from build123d import *

# Parameters (mm, degrees)
BOSS_EXTRUDE1_DEPTH      = 49
CHAMFER1_SIZE            = 1
CHAMFER2_SIZE            = 1
SKETCH4_W                = 3.006754005
SKETCH4_H                = 49
BOSS_EXTRUDE2_DEPTH      = 5
SKETCH5_W                = 49
SKETCH5_H                = 5
BOSS_EXTRUDE3_DEPTH      = 6.139242
BOSS_EXTRUDE4_DEPTH      = 350
BOSS_EXTRUDE4_DEPTH_BACK = 70
SKETCH6_R                = 2.4
BOSS_EXTRUDE5_START      = 50
BOSS_EXTRUDE5_DEPTH      = 50
SKETCH11_R               = 0.5
BOSS_EXTRUDE9_DEPTH      = 2


with BuildPart() as part:
    # Sketch1 → Boss-Extrude1 (new body)
    with BuildSketch(Plane.XY):
        with BuildLine():
            Line((-6.350615501, -38.986147319), (-6.350615501, -41.01121411))
            ThreePointArc((-6.350615501, -41.01121411), (-1.360537007, -41.477692065), (3.649384499, -41.339230675))
            Line((3.649384499, -41.339230675), (3.649384499, -39.331056339))
            ThreePointArc((3.649384499, -39.331056339), (-1.361580989, -39.476525901), (-6.350615501, -38.986147319))
        make_face()
    extrude(amount=BOSS_EXTRUDE1_DEPTH)

    # Chamfer1
    # the kernel refuses this chamfer: 3, 1 mm, written as the material it takes off along each edge
    with BuildSketch(Plane(origin=(3.649384499, -41.339230675, -7.093753287), x_dir=(0, 1, 0), z_dir=(0, 0, 1))) as chamfer1_piece_1:
        with BuildLine():
            Line((CHAMFER1_SIZE, 0), (-0.150364113, 2.720124405))
            ThreePointArc((-0.150364113, 2.720124405), (-0.100586913, 1.415213895), (0, 0))
            Line((0, 0), (CHAMFER1_SIZE, 0))
        make_face()
    extrude(amount=63.187506575, mode=Mode.SUBTRACT)

    # Chamfer2
    # the kernel refuses this chamfer: 3, 1 mm, written as the material it takes off along each edge
    with BuildSketch(Plane(origin=(-6.350615501, -41.01121411, -7.077780992), x_dir=(0.992702552846142, -0.12058872904526673, 0), z_dir=(0, 0, 1))) as chamfer2_piece_1:
        with BuildLine():
            Line((2.717564067, 0), (-CHAMFER2_SIZE * 0.120588729045, CHAMFER2_SIZE * 0.992702552846))
            Line((-CHAMFER2_SIZE * 0.120588729045, CHAMFER2_SIZE * 0.992702552846), (0, 0))
            ThreePointArc((0, 0), (1.415420862, -0.022211756), (2.717564067, 0))
        make_face()
    extrude(amount=63.155561983, mode=Mode.SUBTRACT)

    # Sketch4 → Boss-Extrude2 (add)
    with BuildSketch(Plane(origin=(-17.090415502, -34.725548264, 0), x_dir=(0.8972243095002063, -0.44157506546665215, 0), z_dir=(-0.44157506546665215, -0.8972243095002063, 0))):
        with Locations((13.473404886, 24.5)):
            Rectangle(SKETCH4_W, SKETCH4_H)
    extrude(amount=BOSS_EXTRUDE2_DEPTH)

    # Sketch5 → Boss-Extrude3 (add)
    with BuildSketch(Plane(origin=(-12, 0, 0), x_dir=(0, 0, -1), z_dir=(1, 0, 0))):
        with Locations((-24.5, -45.003805325)):
            Rectangle(SKETCH5_W, SKETCH5_H)
    extrude(amount=BOSS_EXTRUDE3_DEPTH)

    # Sketch6 → Boss-Extrude4 (add, two sides: drawn at the far end of the back side and taken through both)
    with BuildSketch(Plane(origin=(0, 0, 0), x_dir=(-1, 0, 0), z_dir=(0, 0, -1)).offset(-BOSS_EXTRUDE4_DEPTH_BACK)):
        with Locations((12, -45.003805325)):
            Circle(SKETCH6_R)
    extrude(amount=BOSS_EXTRUDE4_DEPTH + BOSS_EXTRUDE4_DEPTH_BACK)

    # Sketch8 → Boss-Extrude5 (add)
    with BuildSketch(Plane(origin=(0, 0, -281.5), x_dir=(-1, 0, 0), z_dir=(0, 0, -1)).offset(BOSS_EXTRUDE5_START)):
        with BuildLine():
            Line((12, -47.503805325), (12, -47.403805325))
            ThreePointArc((12, -47.403805325), (9.6, -45.003805325), (12, -42.603805325))
            Line((12, -42.603805325), (12, -42.503805325))
            Line((12, -42.503805325), (7.577361274, -42.503805325))
            Line((7.577361274, -42.503805325), (6.350615501, -40.01121411))
            Line((6.350615501, -40.01121411), (6.350615501, -38.986147319))
            ThreePointArc((6.350615501, -38.986147319), (1.361580989, -39.476525901), (-3.649384499, -39.331056339))
            Line((-3.649384499, -39.331056339), (-3.649384499, -40.339230675))
            Line((-3.649384499, -40.339230675), (-0.929260095, -41.489594788))
            ThreePointArc((-0.929260095, -41.489594788), (1.363893558, -41.477581829), (3.652882714, -41.338921707))
            Line((3.652882714, -41.338921707), (5.860758041, -45.825043254))
            Line((5.860758041, -45.825043254), (5.860758041, -47.503805325))
            Line((5.860758041, -47.503805325), (12, -47.503805325))
        make_face()
    extrude(amount=-BOSS_EXTRUDE5_DEPTH)

    # Sketch11 → Boss-Extrude9 (add)
    with BuildSketch(Plane(origin=(0, 0, -140.75), x_dir=(-1, 0, 0), z_dir=(0, 0, -1))):
        with BuildLine():
            Line((14.769764267, -46.385196028), (14.147707084, -46.074951572))
            ThreePointArc((14.147707084, -46.074951572), (13.091170315, -47.141408503), (11.607713099, -47.371528068))
            Line((11.607713099, -47.371528068), (14.647174611, -47.875109386))
            ThreePointArc((14.647174611, -47.875109386), (15.517238353, -47.196697988), (14.769764267, -46.385196028))
        make_face()
        with Locations((14.769764267, -47.135196028)):
            Circle(SKETCH11_R, mode=Mode.SUBTRACT)
    extrude(amount=BOSS_EXTRUDE9_DEPTH)


solid = part.part
Source: CAD feature listing. Evaluate the final solid. Frame: model axes, mm. Round coordinates to 2 decimals unless told otherwise and drop trailing zeros. Loops run counter-clockwise (first coordinate to the right, second up) from the corner with the lowest first, then second, coordinate; pieces in that order, holes last.
Q1. Mould query, pull axis X, two halves, no side actions, for faces 1 (the face through (-4, -41, 0)), 2 (the face through (-1.432, -39.474, -306.85)). Classes: pulls with the +X half, pulls with the -X half, needs draft (parallel to the pull), parting line crosses it, or undercut.
Q2. Section B-B, the plane z = -156. Return loops of the section in (x, y), plus the area to 3 significant figures.
Q3. Ray query, line 1 (Z direction, x = -7, y = -45.5); line 2 (X direction, y = -45.25, z = -221.5); line 3 (Y direction, x = -3, z = 46.5). Return the intervals inside material, ascending.
Q4. Section A-A, the plane z = -316. Return loops of the section in (x, y), plus the area to 3 significant figures.
Q5. First-contact query: P1, Ø1.3, axis at y = -47, z = 13.5, coming from the +X side; P2, Ø1.3, axis at x = -10, z = -308, coming from the +Y side; P3, Ø0.8, axis at y = -39.5, z = 34, coming from the -X side. Flat tips, straight axial feed; report the tip coordinate or a pass-through.
Solutions:
1. face 1: needs draft
1. face 2: undercut
2. outline: circle Ø4.8 at (-12, -45)
2. area: 18.1 mm2
3. line 1: z = -331.5 to -281.5, 0 to 49
3. line 2: x = -14.39 to -9.61
3. line 3: y = -41.39 to -39.39
4. outline: (-12, -47.5) - (-5.86, -47.5) - (-5.86, -45.83) - (-3.65, -41.34) arc R41.5 ccw to (0.93, -41.49) - (3.65, -40.34) - (3.65, -39.33) arc R39.5 cw to (-6.35, -38.99) - (-6.35, -40.01) - (-7.58, -42.5) - (-12, -42.5) - (-12, -42.6) arc R2.4 ccw to (-12, -47.4) - close
4. area: 65.9 mm2
5. P1: stops at x = -5.86
5. P2: stops at y = -42.5
5. P3: stops at x = -6.35
